```python
from build123d import *

# Parameters (mm, degrees)
SKETCH1_W               = 110.5662
SKETCH1_H               = 69.342
BOSS_EXTRUDE1_DEPTH     = 9.525
BOSS_EXTRUDE2_DEPTH     = 34.925
BOSS_EXTRUDE3_START     = 34.925
SKETCH1_5_W             = 85.1662
SKETCH1_5_H             = 6.35
SKETCH1_5_W_2           = 6.35
SKETCH1_5_H_2           = 43.942
BOSS_EXTRUDE3_DEPTH     = 4.7625
BOSS_EXTRUDE4_START     = -55.2831
BOSS_EXTRUDE4_DEPTH     = 110.5662
CUT_EXTRUDE3_DEPTH      = 98.551022627
CUT_EXTRUDE3_DEPTH_BACK = 98.551022627
SKETCH1_6_R             = 2.4892
CUT_EXTRUDE1_DEPTH      = 100.785108409
CUT_EXTRUDE1_DEPTH_BACK = 100.785108409
SKETCH3_R               = 2.4892
CUT_EXTRUDE2_DEPTH      = 103.20307776
CUT_EXTRUDE2_DEPTH_BACK = 103.20307776
SKETCH4_R               = 2.4892
FILLET1_R               = 3.175
FILLET2_R               = 3.175


with BuildPart() as part:
    # Sketch1 → Boss-Extrude1 (new, symmetric)
    with BuildSketch(Plane.XY):
        Rectangle(SKETCH1_W, SKETCH1_H)
    extrude(amount=BOSS_EXTRUDE1_DEPTH, both=True)

    # Sketch1<3> → Boss-Extrude2 (add)
    with BuildSketch(Plane.XY):
        Polygon((-55.2831, 21.971), (-48.9331, 21.971), (-48.9331, 28.321), (-42.5831, 28.321), (-42.5831, 34.671), (-55.2831, 34.671), align=None)
        Polygon((48.9331, 28.321), (48.9331, 21.971), (55.2831, 21.971), (55.2831, 34.671), (42.5831, 34.671), (42.5831, 28.321), align=None)
        Polygon((-42.5831, -28.321), (-48.9331, -28.321), (-48.9331, -21.971), (-55.2831, -21.971), (-55.2831, -34.671), (-42.5831, -34.671), align=None)
        Polygon((48.9331, -28.321), (42.5831, -28.321), (42.5831, -34.671), (55.2831, -34.671), (55.2831, -21.971), (48.9331, -21.971), align=None)
    extrude(amount=BOSS_EXTRUDE2_DEPTH)

    # Sketch1<5> → Boss-Extrude3 (add)
    with BuildSketch(Plane.XY.offset(BOSS_EXTRUDE3_START)):
        with Locations((0, 31.496)):
            Rectangle(SKETCH1_5_W, SKETCH1_5_H)
        Polygon((48.9331, 28.321), (48.9331, 21.971), (55.2831, 21.971), (55.2831, 34.671), (42.5831, 34.671), (42.5831, 28.321), align=None)
        with Locations((52.1081, 0)):
            Rectangle(SKETCH1_5_W_2, SKETCH1_5_H_2)
        Polygon((48.9331, -28.321), (42.5831, -28.321), (42.5831, -34.671), (55.2831, -34.671), (55.2831, -21.971), (48.9331, -21.971), align=None)
        with Locations((0, -31.496)):
            Rectangle(SKETCH1_5_W, SKETCH1_5_H)
        Polygon((-42.5831, -28.321), (-48.9331, -28.321), (-48.9331, -21.971), (-55.2831, -21.971), (-55.2831, -34.671), (-42.5831, -34.671), align=None)
        with Locations((-52.1081, 0)):
            Rectangle(SKETCH1_5_W_2, SKETCH1_5_H_2)
        Polygon((-55.2831, 21.971), (-48.9331, 21.971), (-48.9331, 28.321), (-42.5831, 28.321), (-42.5831, 34.671), (-55.2831, 34.671), align=None)
    extrude(amount=BOSS_EXTRUDE3_DEPTH)

    # Sketch2 → Boss-Extrude4 (add)
    with BuildSketch(Plane(origin=(0, 0, 0), x_dir=(0, 0, -1), z_dir=(1, 0, 0)).offset(BOSS_EXTRUDE4_START)):
        Polygon((9.525, 34.671), (9.525, -34.671), (25.914946669, -58.078269666), (28.515754409, -56.25716448), (13.946912926, -35.450702555), (55.559836776, -6.313019589), (53.73873159, -3.712211848), (42.105082855, -11.858180389), align=None)
    extrude(amount=BOSS_EXTRUDE4_DEPTH)

    # Sketch1<6> → Cut-Extrude3 (cut, two sides: drawn at the far end of the back side and taken through both)
    with BuildSketch(Plane.XY.offset(-CUT_EXTRUDE3_DEPTH_BACK)):
        with Locations((-44.4246, 23.8125)):
            Circle(SKETCH1_6_R)
        with Locations((44.4246, 23.8125)):
            Circle(SKETCH1_6_R)
        with Locations((44.4246, -23.8125)):
            Circle(SKETCH1_6_R)
        with Locations((-44.4246, -23.8125)):
            Circle(SKETCH1_6_R)
    extrude(amount=CUT_EXTRUDE3_DEPTH + CUT_EXTRUDE3_DEPTH_BACK, mode=Mode.SUBTRACT)

    # Sketch3 → Cut-Extrude1 (cut, two sides: drawn at the far end of the back side and taken through both)
    with BuildSketch(Plane(origin=(0, -6.931123699, 9.898670495), x_dir=(1, 0, 0), z_dir=(0, -0.5735764363510447, 0.8191520442889929)).offset(-CUT_EXTRUDE1_DEPTH_BACK)):
        with Locations(Location((-48.9331, -56.089136084, 0), (0, 0, 270))):
            Circle(SKETCH3_R)
        with Locations(Location((-34.952214286, -56.089136084, 0), (0, 0, 270))):
            Circle(SKETCH3_R)
        with Locations(Location((-20.971328571, -56.089136084, 0), (0, 0, 270))):
            Circle(SKETCH3_R)
        with Locations(Location((-6.990442857, -56.089136084, 0), (0, 0, 270))):
            Circle(SKETCH3_R)
        with Locations(Location((6.990442857, -56.089136084, 0), (0, 0, 270))):
            Circle(SKETCH3_R)
        with Locations(Location((20.971328571, -56.089136084, 0), (0, 0, 270))):
            Circle(SKETCH3_R)
        with Locations(Location((34.952214286, -56.089136084, 0), (0, 0, 270))):
            Circle(SKETCH3_R)
        with Locations(Location((48.9331, -56.089136084, 0), (0, 0, 270))):
            Circle(SKETCH3_R)
        with Locations(Location((-34.952214286, -43.389136084, 0), (0, 0, 270))):
            Circle(SKETCH3_R)
        with Locations(Location((-20.971328571, -43.389136084, 0), (0, 0, 270))):
            Circle(SKETCH3_R)
        with Locations(Location((-6.990442857, -43.389136084, 0), (0, 0, 270))):
            Circle(SKETCH3_R)
        with Locations(Location((6.990442857, -43.389136084, 0), (0, 0, 270))):
            Circle(SKETCH3_R)
        with Locations(Location((20.971328571, -43.389136084, 0), (0, 0, 270))):
            Circle(SKETCH3_R)
        with Locations(Location((34.952214286, -43.389136084, 0), (0, 0, 270))):
            Circle(SKETCH3_R)
        with Locations(Location((48.9331, -43.389136084, 0), (0, 0, 270))):
            Circle(SKETCH3_R)
        with Locations(Location((-48.9331, -43.389136084, 0), (0, 0, 270))):
            Circle(SKETCH3_R)
    extrude(amount=CUT_EXTRUDE1_DEPTH + CUT_EXTRUDE1_DEPTH_BACK, mode=Mode.SUBTRACT)

    # Sketch4 → Cut-Extrude2 (cut, two sides: drawn at the far end of the back side and taken through both)
    with BuildSketch(Plane(origin=(0, -27.739876301, -19.423670495), x_dir=(1, 0, 0), z_dir=(0, 0.8191520442889928, 0.5735764363510449)).offset(-CUT_EXTRUDE2_DEPTH_BACK)):
        with Locations(Location((48.9331, 35.540954597, 0), (0, 0, 270))):
            Circle(SKETCH4_R)
        with Locations(Location((34.952214286, 35.540954597, 0), (0, 0, 270))):
            Circle(SKETCH4_R)
        with Locations(Location((20.971328571, 35.540954597, 0), (0, 0, 270))):
            Circle(SKETCH4_R)
        with Locations(Location((6.990442857, 35.540954597, 0), (0, 0, 270))):
            Circle(SKETCH4_R)
        with Locations(Location((-6.990442857, 35.540954597, 0), (0, 0, 270))):
            Circle(SKETCH4_R)
        with Locations(Location((-20.971328571, 35.540954597, 0), (0, 0, 270))):
            Circle(SKETCH4_R)
        with Locations(Location((-34.952214286, 35.540954597, 0), (0, 0, 270))):
            Circle(SKETCH4_R)
        with Locations(Location((-48.9331, 35.540954597, 0), (0, 0, 270))):
            Circle(SKETCH4_R)
    extrude(amount=CUT_EXTRUDE2_DEPTH + CUT_EXTRUDE2_DEPTH_BACK, mode=Mode.SUBTRACT)

    # Fillet1
    fillet1_edges = [part.edges().sort_by_distance(p)[0] for p in [
        (0, -11.858180389, -42.105082855),
        (0, 34.671, -9.525),
        (0, -34.671, -9.525),
    ]]
    fillet(fillet1_edges, radius=FILLET1_R)

    # Fillet2
    fillet2_edges = [part.edges().sort_by_distance(p)[0] for p in [
        (48.9331, -28.321, 24.60625),
        (42.5831, -28.321, 22.225),
        (-42.5831, -28.321, 22.225),
        (-48.9331, -28.321, 24.60625),
        (-48.9331, 21.971, 22.225),
        (-48.9331, 28.321, 24.60625),
        (-42.5831, 28.321, 22.225),
        (42.5831, 28.321, 22.225),
        (48.9331, 28.321, 24.60625),
        (48.9331, 21.971, 22.225),
        (48.9331, -21.971, 22.225),
        (-48.9331, -21.971, 22.225),
        (55.2831, 21.971, 22.225),
        (-42.5831, -34.671, 22.225),
        (42.5831, -34.671, 22.225),
        (55.2831, -21.971, 22.225),
        (-55.2831, -21.971, 22.225),
        (-55.2831, 21.971, 22.225),
        (-42.5831, 34.671, 22.225),
        (42.5831, 34.671, 22.225),
    ]]
    fillet(fillet2_edges, radius=FILLET2_R - 0.0001)  # a hair under: the kernel refuses the full size


solid = part.part
```
Could you check a few things on this model? Use its own coordinates, in mm. A direction names the side the tool comes from. Coordinates: 2 decimals unless noted, no trailing zeros. Loops run counter-clockwise (first coordinate to the right, second up) from the corner with the lowest first, then second, coordinate; pieces in that order, holes last.
1) Will these pins go through, and if not, where does the flat tip stop? pin 1 Ø1 at (x, z) = (-41, 17) entering from -Y; pin 2 Ø1.5 at (x, y) = (6, -9) entering from -Z; pin 3 Ø12 at (x, y) = (37.5, -39.5) entering from -Z; pin 4 Ø5.5 at (x, y) = (-44.42, -23.81) entering from -Z.
Reported:
pin 1: passes through
pin 2: stops at z = -52.79
pin 3: stops at z = -20.98
pin 4: stops at z = -34.5
2) Imagine slicing it at C-C (z = -32.5). List the corners of the cut face in (x, y) for me.
Reported:
outline: (-55.28, -22.46) - (-46.51, -22.46) arc R2.49 cw to (-42.34, -22.46) - (42.34, -22.46) arc R2.49 cw to (46.51, -22.46) - (55.28, -22.46) - (55.28, 1.86) - (-55.28, 1.86) - close
3) Thinking about a two-plate mould opening in X: for faces 1 (the face through (0.77, -35.04, -9.36)), 2 (the face through (-54.38, 22.93, 22.4)), 3 (the face through (44.101, -21.344, -12.605)), which applies, released by +X, released by -X, zero draft, split by the parting line, or undercut?
Reported:
face 1: zero draft
face 2: released by -X
face 3: undercut
4) Imagine slicing it at B-B (z = 16). State how many separate pieces and enclosed holes the cut face has, and give its area (3 significant figures).
Reported:
separate pieces: 4
enclosed holes: 0
area: 458 mm2
5) Please list where these lines run through material, in increasing order: line 1 along Y through (x, z) = (-42.5, 0); line 2 along Y through (x, z) = (1.5, 2); line 3 along Z through (x, y) = (17.5, 28.5) (1 decimal).
Reported:
line 1: y = -34.67 to -25.39, -22.23 to 22.23, 25.39 to 34.67
line 2: y = -34.67 to 34.67
line 3: z = -13.8 to 9.5, 34.9 to 39.7
6) Which directions (+Z, -Z, +X, -X, +Y, -Y) give clear straight access to the entire face, cutting with the end or side of a thin tool? Please do faces 4 (the face through (-48.933, 0, 37)), 5 (the face through (-0.77, -46.9, -18.09)), 6 (the face through (-1, 0, 9.525)).
Reported:
face 4: +Z
face 5: +Z, +X, -X, -Y
face 6: none
7) Imagine slicing it at A-A (y = -19). List the corners of the cut face in (x, z) for me (1 decimal), and give its area (3 significant figures).
Reported:
outline: (-55.3, -37.4) - (55.3, -37.4) - (55.3, 9.5) - (-55.3, 9.5) - close; (-55.3, 34.9) - (-48.9, 34.9) - (-48.9, 39.7) - (-55.3, 39.7) - close; (48.9, 34.9) - (55.3, 34.9) - (55.3, 39.7) - (48.9, 39.7) - close
area: 5,250 mm2
8) Imagine slicing it at D-D (y = 18.5). List the corners of the cut face in (x, z) for me (1 decimal), and give its area (3 significant figures).
Reported:
outline: (-55.3, -20.8) - (55.3, -20.8) - (55.3, 9.5) - (-55.3, 9.5) - close; (-55.3, 34.9) - (-48.9, 34.9) - (-48.9, 39.7) - (-55.3, 39.7) - close; (48.9, 34.9) - (55.3, 34.9) - (55.3, 39.7) - (48.9, 39.7) - close
area: 3,420 mm2
